Check sheet for the modelled part. Datum: model origin and axes. Units: mm. A direction names the side the tool comes from. Give positions to 0.01 mm unless a question says otherwise; leave off trailing zeros. Order: outer loops, then holes, each group sorted by start corner. A loop starts at its lowest first (then second) coordinate and runs counter-clockwise, first axis right, second up. Notation, with made-up numbers: (71.25, 38.25) -> (97.25, 38.25) arc R21 cw to (97.25, 69.25) -> close; hole circle Ø5 at (13, 73). An arc over 180 degrees is marked (long way). One line per question, with ' | ' between items.
```python
from build123d import *

# Parameters (mm, degrees)
SKETCH1_W           = 12.8
SKETCH1_H           = 6.8
BOSS_EXTRUDE1_DEPTH = 6.5
BOSS_EXTRUDE2_DEPTH = 0.3
SKETCH3_W           = 3.9
SKETCH3_H           = 3.9
BOSS_EXTRUDE3_DEPTH = 5.08
SKETCH4_W           = 1
SKETCH4_H           = 2
BOSS_EXTRUDE4_DEPTH = 4
CUT_EXTRUDE1_DEPTH  = 20.471384132


with BuildPart() as part:
    # Sketch1 → Boss-Extrude1 (new body)
    with BuildSketch(Plane(origin=(0, 0, 0), x_dir=(1, 0, 0), z_dir=(0, 1, 0))):
        Rectangle(SKETCH1_W, SKETCH1_H)
    extrude(amount=BOSS_EXTRUDE1_DEPTH)

    # Sketch2 → Boss-Extrude2 (add)
    with BuildSketch(Plane(origin=(0, 6.5, 0), x_dir=(1, 0, 0), z_dir=(0, 1, 0))):
        with BuildLine():
            Line((9.78, 3.05), (-9.78, 3.05))
            Line((-9.78, 3.05), (-9.78, 1.5))
            Line((-9.78, 1.5), (-8.765, 1.5))
            ThreePointArc((-8.765, 1.5), (-7.265, 0), (-8.765, -1.5))
            Line((-8.765, -1.5), (-9.78, -1.5))
            Line((-9.78, -1.5), (-9.78, -3.05))
            Line((-9.78, -3.05), (9.78, -3.05))
            Line((9.78, -3.05), (9.78, -1.5))
            Line((9.78, -1.5), (8.765, -1.5))
            ThreePointArc((8.765, -1.5), (7.265, 0), (8.765, 1.5))
            Line((8.765, 1.5), (9.78, 1.5))
            Line((9.78, 1.5), (9.78, 3.05))
        make_face()
    extrude(amount=-BOSS_EXTRUDE2_DEPTH)

    # Sketch3 → Boss-Extrude3 (add)
    with BuildSketch(Plane(origin=(0, 6.5, 0), x_dir=(1, 0, 0), z_dir=(0, 1, 0))):
        Rectangle(SKETCH3_W, SKETCH3_H)
    extrude(amount=BOSS_EXTRUDE3_DEPTH)

    # Sketch4 → Boss-Extrude4 (add)
    with BuildSketch(Plane.XZ):
        Rectangle(SKETCH4_W, SKETCH4_H)
        with Locations((5, 0)):
            Rectangle(SKETCH4_W, SKETCH4_H)
        with Locations((-5, 0)):
            Rectangle(SKETCH4_W, SKETCH4_H)
    extrude(amount=BOSS_EXTRUDE4_DEPTH)

    # Sketch5 → Cut-Extrude1 (cut, through all)
    with BuildSketch(Plane(origin=(5.5, 0, 0), x_dir=(0, 0, -1), z_dir=(1, 0, 0))):
        with BuildLine():
            Line((0.595, -1.01), (0.595, -2.99))
            ThreePointArc((0.595, -2.99), (0, -3.585), (-0.595, -2.99))
            Line((-0.595, -2.99), (-0.595, -1.01))
            ThreePointArc((-0.595, -1.01), (0, -0.415), (0.595, -1.01))
        make_face()
    extrude(amount=-CUT_EXTRUDE1_DEPTH, mode=Mode.SUBTRACT)


solid = part.part
```
Q1. Section check A-A (x = -4.75). Enter the section's corners in (y, z) (3 decimals).
Result sheet:
outline: (-4, -1) -> (0, -1) -> (0, -3.4) -> (6.5, -3.4) -> (6.5, 3.4) -> (0, 3.4) -> (0, 1) -> (-4, 1) -> close; hole (-2.99, -0.595) -> (-1.01, -0.595) arc R0.595 ccw to (-1.01, 0.595) -> (-2.99, 0.595) arc R0.595 ccw to start
Q2. Section check C-C (z = 0). Count the separate pieces of the cut face and the enclosed holes in it, and give its area (3 significant figures).
Result sheet:
separate pieces: 4 | enclosed holes: 0 | area: 106 mm2
Q3. Section check B-B (x = 7.75). Enter the section's corners in (y, z).
Result sheet:
outline: (6.2, -3.05) -> (6.5, -3.05) -> (6.5, -1.1) -> (6.2, -1.1) -> close; (6.2, 1.1) -> (6.5, 1.1) -> (6.5, 3.05) -> (6.2, 3.05) -> close
Q4. Mould release check, pull along Z, two halves, no side actions. Record for faces 1 (the face through (5.007, -0.415, 0.013)), 2 (the face through (0, 3, 3.4)), 3 (the face through (0, 11.58, 0)): pulls with the +Z half, pulls with the -Z half, needs draft (parallel to the pull), parting line crosses it, or undercut.
Result sheet:
face 1: undercut | face 2: pulls with the +Z half | face 3: needs draft
Q5. Section check D-D (y = 7.75). Enter the section's corners in (x, z).
Result sheet:
outline: (-1.95, -1.95) -> (1.95, -1.95) -> (1.95, 1.95) -> (-1.95, 1.95) -> close
Q6. Thickness scan on line 1 (X direction, y = 0.5, z = -2.75); line 2 (Y direction, x = -3.5, z = 0.25); line 3 (Z direction, x = 1, y = 8). Record the ranges inside material, lowest first.
Result sheet:
line 1: x = -6.4 to 6.4 | line 2: y = 0 to 6.5 | line 3: z = -1.95 to 1.95
Q7. Depth check by flat-ended pin: pin 1 Ø2 at (y, z) = (10, -0.5) entering from +X; pin 2 Ø1.1 at (x, y) = (5, -1.5) entering from +Z; pin 3 Ø1.5 at (x, z) = (-6.5, 0) entering from -Y; pin 4 Ø1 at (y, z) = (-2.5, 0) entering from +X. Enter the tip coordinate at first touch or a pass-through.
Result sheet:
pin 1: stops at x = 1.95 | pin 2: stops at z = 1 | pin 3: stops at y = 0 | pin 4: passes through
Q8. Access from +Z, -Z, +X, -X, +Y, -Y to the whole of each face (thin tool, end or side, straight path). Record for faces 4 (the face through (5, -2, 0.595)), 5 (the face through (1.95, 9, 0)), 6 (the face through (0, -2, 1)).
Result sheet:
face 4: +X, -X | face 5: +Z, -Z, +X, +Y | face 6: +Z, +X, -X, -Y
